from build123d import *

# Parameters (mm, degrees)
SKETCH2_W               = 58
SKETCH2_H               = 4
BOSS_EXTRUDE1_DEPTH     = 5
CUT_EXTRUDE4_START      = -2
CUT_EXTRUDE4_DEPTH      = 4
CUT_EXTRUDE8_DEPTH      = 30.495762408
CUT_EXTRUDE8_DEPTH_BACK = 30.495762408
SKETCH4_R               = 1.5
BOSS_EXTRUDE2_DEPTH     = 5
SKETCH6_R               = 25.176714318
CUT_EXTRUDE7_DEPTH      = 48.546713727
SKETCH8_R               = 2
CUT_EXTRUDE9_DEPTH      = 46.466564837
FILLET1_R               = 2


# Read off the part's stored shape, not the designer's step: Cut-Extrude4
with BuildPart() as part:
    # Sketch2 → Boss-Extrude1 (new, symmetric)
    with BuildSketch(Plane(origin=(0, 0, 0), x_dir=(1, 0, 0), z_dir=(0, 1, 0))):
        Rectangle(SKETCH2_W, SKETCH2_H)
    extrude(amount=BOSS_EXTRUDE1_DEPTH, both=True)

    # Cut-Extrude4 outline → Cut-Extrude4 (cut)
    with BuildSketch(Plane.XY.offset(CUT_EXTRUDE4_START)):
        with BuildLine():
            ThreePointArc((-29, 2.66e-07), (-28.891224415, 2.509412642), (-28.565713714, 5))
            Line((-28.565713714, 5), (-29, 5))
            Line((-29, 5), (-29, 2.66e-07))
        make_face()
        with BuildLine():
            ThreePointArc((-28.565713714, -5), (-28.891224438, -2.509412377), (-29, 2.66e-07))
            Line((-29, 2.66e-07), (-29, -5))
            Line((-29, -5), (-28.565713714, -5))
        make_face()
        with BuildLine():
            Line((29, 5), (28.565713714, 5))
            ThreePointArc((28.565713714, 5), (28.891224438, 2.509412377), (29, -2.66e-07))
            Line((29, -2.66e-07), (29, 5))
        make_face()
        with BuildLine():
            Line((29, -5), (29, -2.66e-07))
            ThreePointArc((29, -2.66e-07), (28.891224415, -2.509412642), (28.565713714, -5))
            Line((28.565713714, -5), (29, -5))
        make_face()
    extrude(amount=CUT_EXTRUDE4_DEPTH, mode=Mode.SUBTRACT)

    # Sketch4 → Cut-Extrude8 (cut, two sides: drawn at the far end of the back side and taken through both)
    with BuildSketch(Plane.XY.offset(-CUT_EXTRUDE8_DEPTH_BACK)):
        with Locations((16, 0)):
            Circle(SKETCH4_R)
        with Locations((-16, 0)):
            Circle(SKETCH4_R)
    extrude(amount=CUT_EXTRUDE8_DEPTH + CUT_EXTRUDE8_DEPTH_BACK, mode=Mode.SUBTRACT)

    # Sketch5 → Boss-Extrude2 (add, symmetric)
    with BuildSketch(Plane(origin=(0, 0, 0), x_dir=(1, 0, 0), z_dir=(0, 1, 0))):
        with BuildLine():
            Line((-24, -17), (-24.675229358, -18.882568807))
            ThreePointArc((-24.675229358, -18.882568807), (-29.952612974, 20.143186858), (5, 2))
            Line((5, 2), (3, 2))
            ThreePointArc((3, 2), (-28.801626162, 18.507574019), (-24, -17))
        make_face()
        with BuildLine():
            Line((-3, 2), (-5, 2))
            ThreePointArc((-5, 2), (29.952612974, 20.143186858), (24.675229358, -18.882568807))
            Line((24.675229358, -18.882568807), (24, -17))
            ThreePointArc((24, -17), (28.801626162, 18.507574019), (-3, 2))
        make_face()
    extrude(amount=BOSS_EXTRUDE2_DEPTH, both=True)

    # Sketch6 → Cut-Extrude7 (cut, through all)
    with BuildSketch(Plane.XY.offset(2)):
        Circle(SKETCH6_R)
    extrude(amount=CUT_EXTRUDE7_DEPTH, mode=Mode.SUBTRACT)

    # Sketch8 → Cut-Extrude9 (cut, through all)
    with BuildSketch(Plane(origin=(0, 0, -2), x_dir=(-1, 0, 0), z_dir=(0, 0, -1))):
        with Locations(Location((16, 0, 0), (0, 0, 180))):
            Circle(SKETCH8_R)
        with Locations(Location((-16, 0, 0), (0, 0, 180))):
            Circle(SKETCH8_R)
    extrude(amount=CUT_EXTRUDE9_DEPTH, mode=Mode.SUBTRACT)

    # Fillet1
    fillet1_edges = [part.edges().sort_by_distance(p)[0] for p in [
        (0, 0, -16.030390296),
        (0, 0, -12.58825345),
        (3, 0, -2),
        (5, 0, -2),
        (-5, 0, -2),
        (-3, 0, -2),
        (-1.232758621, 0, -14.367772138),
        (1.232758621, 0, -14.367772138),
    ]]
    fillet(fillet1_edges, radius=FILLET1_R)


solid = part.part
Can you work these out from the model? Positions are in its coordinate system, mm. A direction names the side the tool comes from. Give positions to 0.01 mm unless a question says otherwise; leave off trailing zeros. Order: outer loops, then holes, each group sorted by start corner. A loop starts at its lowest first (then second) coordinate and runs counter-clockwise, first axis right, second up. Notation, with made-up numbers: M 80,85 L 118,85 A21 ccw 118,105 Z; hole C 16,23 d2. An arc over 180 degrees is marked long. One line per item, written item: value.
Item 1: If we section it at B-B on x = -8.5: Write out the boundary of the cut face in (y, z).
Verdict:
outline: M -5,-22.41 L 5,-22.41 L 5,-20.22 L -5,-20.22 Z; M -5,-2 L 5,-2 L 5,2 L -5,2 Z
Item 2: If we section it at D-D on y = 0.75: State how many separate pieces and enclosed holes the cut face has, and give its area (3 significant figures).
Verdict:
separate pieces: 5
enclosed holes: 1
area: 569 mm2
Item 3: If we mould it in two halves opening along X, with no side actions, what happens to faces 1 (the face through (-3, 5, -8)), 2 (the face through (-33.46, 0.07, -13.94)), 3 (the face through (2.364, -0.07, -2.648))? For each: pulls with the +X half, pulls with the -X half, needs draft (parallel to the pull), parting line crosses it, or undercut.
Verdict:
face 1: needs draft
face 2: undercut
face 3: undercut
Item 4: If we section it at A-A on z = -7.5: Write out the boundary of the cut face in (x, y), and give its area (3 significant figures).
Verdict:
outline: M -38.68,-5 L -36.61,-5 L -36.61,5 L -38.68,5 Z; M -4.31,-5 L -2.24,-5 L -2.24,5 L -4.31,5 Z; M 2.24,-5 L 4.31,-5 L 4.31,5 L 2.24,5 Z; M 36.61,-5 L 38.68,-5 L 38.68,5 L 36.61,5 Z
area: 82.8 mm2
Item 5: If we section it at C-C on z = 10: Write out the boundary of the cut face in (x, y).
Verdict:
outline: M -35.84,-5 L -33.42,-5 L -33.42,5 L -35.84,5 Z; M 33.42,-5 L 35.84,-5 L 35.84,5 L 33.42,5 Z
Item 6: For pin 1 (3.5 mm diameter, centred on x = -16, y = 0, fed in from -Z); pin 2 (3 mm diameter, centred on x = -22.5, y = 1.5, fed in from -Z); pin 3 (6 mm diameter, centred on x = -10, y = 1.5, fed in from +Z), each with a flat end and sliding along its axis, tell me the tip position at first contact or that it passes through.
Verdict:
pin 1: z = -2
pin 2: z = -23.85
pin 3: z = 2
Item 7: Please list where these lines run through material, in increasing order: line 1 (Z direction, x = 26, y = -3.5); line 2 (X direction, y = 0.25, z = -3.5); line 3 (Y direction, x = 16, z = -23.2).
Verdict:
line 1: -22.36 to -20.16, -2 to 2, 16.16 to 18.36
line 2: -39.32 to -37.31, -4.98 to -2.83, 2.83 to 4.98, 37.31 to 39.32
line 3: -5 to -2, 2 to 5
Item 8: For faces 4 (the face through (-17.5, 0.07, -0.03)), 5 (the face through (25.177, -0.07, 17.693)), 6 (the face through (-17.6, 1.2, -23)), 7 (the face through (18, 0, -2)), which set-ups out of +Z, -Z, +X, -X, +Y, -Y let a thin tool reach every point of the face, with its end or its side?
Verdict:
face 4: +Z, -Z
face 5: +Z
face 6: -Z
face 7: +Y, -Y
